Autodesk Fusion 360 part; units mm, degrees
sketch "スケッチ1" plane through (0, 0, 0) normal (0, 0, 1) x (1, 0, 0)
  line L0 (0, 0) -> (18.0857, 0)
  line L1 (18.0857, 0) -> (18.0857, 13.2439)
  line L2 (18.0857, 13.2439) -> (0, 13.2439)
  line L3 (0, 13.2439) -> (0, 0)
  line L4 (0, 0) -> (-13.9996, 0)
  line L5 (-13.9996, 0) -> (-13.9996, 13.2439)
  line L6 (-13.9996, 13.2439) -> (0, 13.2439)
  line L7 (0, 13.2439) -> (0, 0)
  circle A0 centre (-6.9857, 4.9) radius 2
  circle A1 centre (6.9857, 4.9) radius 2
  circle A2 centre (0, 9) radius 2
  circle A3 centre (14.1857, 2.8) radius 3
  circle A4 centre (-6.9857, 4.9) radius 2.5
  circle A5 centre (6.9857, 4.9) radius 2.5
  circle A6 centre (0, 9) radius 2.3
  circle A7 centre (0, 9) radius 1.7
  line L8 (-7, 1.5) -> (-7, 0)
  line L9 (7, 1.5) -> (7, 0)
  circle A8 centre (-6.9857, 4.9) radius 3.4
  circle A9 centre (0, 9) radius 2.9
  line L10 (-6.9857, 4.9) -> (0, 9)
  line L11 (0, 9) -> (6.9857, 4.9)
  line L12 (6.9857, 4.9) -> (14.1857, 2.8)
  circle A10 centre (6.9857, 4.9) radius 3.4
  circle A11 centre (14.1857, 2.8) radius 3.9
  line L13 (-4.6, 2.4775) -> (-4.6, 0)
  line L14 (4.6, 2.4775) -> (4.6, 0)
  line L15 (-9.4, 2.506) -> (-9.4, 0)
  line L16 (9.4, 2.506) -> (9.4, 0)
  line L17 (-3.6347, 5.4753) -> (-1.6695, 6.6287)
  line L18 (1.6695, 6.6287) -> (3.6347, 5.4753)
  line L19 (-4.8495, 7.5452) -> (-2.8843, 8.6986)
  line L20 (2.8843, 8.6986) -> (4.8495, 7.5452)
  line L21 (10.2588, 5.8204) -> (11.3683, 5.4967)
  line L22 (9.2508, 2.3644) -> (10.3603, 2.0407)
  line L23 (0, 0) -> (18.0857, 0)
  line L24 (18.0857, 0) -> (18.0857, -2.0683)
  line L25 (18.0857, -2.0683) -> (0, -2.0683)
  line L26 (-13.9996, 0) -> (0, 0)
  line L27 (0, -2.0683) -> (-13.9996, -2.0683)
  line L28 (-13.9996, -2.0683) -> (-13.9996, 0)
  line L29 (-12.3, 6.4) -> (-12.3, 10)
  line L30 (-12.3, 10) -> (-8.7, 10)
  line L31 (-8.7, 10) -> (-8.7, 7.8362)
  line L32 (-12.3, 6.4) -> (-10.0369, 6.4)
  line L33 (-5.5, 1.65) -> (-8.5, 1.65)
  line L34 (-8.5, 1.65) -> (-8.5, 0.4)
  line L35 (-8.5, 0.4) -> (-5.5, 0.4)
  line L36 (-5.5, 0.4) -> (-5.5, 1.65)
  line L37 (-5.5, 1.65) -> (-8.5, 0.4) construction
  line L38 (-8.5, 1.65) -> (-5.5, 0.4) construction
  line L39 (8.5, 1.65) -> (5.5, 1.65)
  line L40 (5.5, 1.65) -> (5.5, 0.4)
  line L41 (5.5, 0.4) -> (8.5, 0.4)
  line L42 (8.5, 0.4) -> (8.5, 1.65)
  line L43 (8.5, 1.65) -> (5.5, 0.4) construction
  line L44 (5.5, 1.65) -> (8.5, 0.4) construction
  arc A12 (-12.3, 9.4) -> (-9.3, 6.4) centre (-9.3, 9.4) ccw
  point P0 (-7, 1.5)
  point P1 (7, 1.5)
  point P2 (-10.5, 10)
  point P3 (-7, 1.025)
  point P4 (7, 1.025)
  dimension "d4" = 4
  dimension "d5" = 4.9
  dimension "d6" = 8.1
  dimension "d7" = 4
  dimension "d10" = 6
  dimension "d16" = 2.8
  dimension "d18" = 9
  dimension "d19" = 5
  dimension "d21" = 7.5
  dimension "d26" = 4.6
  dimension "d34" = 3.4
  dimension "d41" = 7
  dimension "d45" = 5.8
  dimension "d51" = 1.2
  dimension "d52" = 4.8
  dimension "d54" = 1.8
  dimension "d57" = 6.8
  dimension "d76" = 7.8
  dimension "d86" = 10.5
  dimension "d87" = 3.6
  dimension "d88" = 10
  dimension "d92" = 3
  dimension "d93" = 0.4
  dimension "d94" = 1.25
  dimension "d96" = 3.6
  dimension "d97" = 3
extrude "押し出し1" add sketch "スケッチ1" along normal blind 3 contours L0 L9 A10 L14 L23 L39 L40 L41 | L3 L7 A6 A9 L10 | L3 L7 A6 A9 L11 | L4 L8 A8 L13 L26 L33 L35 L36 | L0 L9 A10 L16 L22 L23 L39 L41 L42 | A5 L11 L12 A10 L39 | A8 A9 L10 L17 | A9 L11 A10 L18 | L4 L8 A8 L15 L26 L33 L34 L35 | A8 L33 | L3 L7 A6 A9 L10 | L3 L7 A6 A9 L11 | A8 A9 L10 L19 | A9 L11 A10 L20 | L0 A3 L12 A11 L23 | L0 A3 A11 L23 | A10 L16 L22 | L12 A10 A11 L16 L22 | A5 L11 L12 A10 | L0 A3 L12 A11 L23 | L12 A10 A11 L21 | A8 L29 L30 L31 A12 picked at (-7.0288, 1.9011)
extrude "押し出し2" add sketch "スケッチ1" along normal blind 0.5 contours A4 | A1 A5 L11 L12 | A1 A5 L11 L12
extrude "押し出し5" add sketch "スケッチ1" against normal blind 2.3 from surface at 3 contours L3 L7 A2 A6 L10 | L3 L7 A2 A6 L11 | L3 L7 A2 A6 L10 | L3 L7 A2 A6 L11
sketch "スケッチ2" plane through (0, 0, 0) normal (0, -1, 0) x (1, 0, 0)
  line L0 (-7, 0) -> (-7, 3)
  line L1 (7, 0) -> (7, 3)
  circle A0 centre (-7, 1.5) radius 0.8
  circle A1 centre (7, 1.5) radius 0.8
  line L2 (9.4, 0) -> (9.4, 3)
  line L3 (4.6, 3) -> (4.6, 0)
  line L4 (-4.6, 3) -> (-9.4, 3)
  line L5 (4.6, 0) -> (9.4, 0)
  line L6 (-4.6, 0) -> (-4.6, 3)
  line L7 (-9.4, 3) -> (-9.4, 0)
  line L8 (9.4, 3) -> (4.6, 3)
  line L9 (-9.4, 0) -> (-4.6, 0)
  point P0 (7, 0)
  dimension "d42" = 1.6
extrude "押し出し7" cut sketch "スケッチ2" against normal blind 3 contours L0 A0 | L0 A0 | L1 A1 | L1 A1
extrude "押し出し8" add sketch "スケッチ1" against normal blind 0.3 from surface at 1 contours L3 L7 A2 A7 L10 | L3 L7 A2 A7 L11 | L3 L7 A2 A7 L10 | L3 L7 A2 A7 L11
sketch "スケッチ6" plane through (0, 10, 0) normal (0, 1, 0) x (-1, 0, 0)
  line L0 (8.7, 0) -> (12.3, 0)
  line L1 (12.3, 0) -> (12.3, 3)
  line L2 (12.3, 3) -> (8.7, 3)
  line L3 (8.7, 3) -> (8.7, 0)
  line L4 (10.5, 3) -> (10.5, 0)
  circle A0 centre (10.5, 1.5) radius 0.75
  dimension "d89" = 1.5
extrude "押し出し12" cut sketch "スケッチ6" against normal blind 2.6 contours L4 A0 | L4 A0
equation "d5 = 6.5 mm - 0.6 mm - 1.0 mm"
equation "d6 = 6 mm + 2.0 mm + 0.1 mm"
equation "d16 = ( 7.8 / 2 ) * 1 mm - 0.6 mm - 0.5 mm"
equation "d21 = 6 mm + 1.4 mm + 0.1 mm"
Input: part model. Units: mm. Frame: model coordinates. A direction names the side the tool comes from. Coordinates: 2 decimals unless noted, no trailing zeros. Write each loop counter-clockwise with the first axis right and the second up, starting at its lowest first coordinate (ties: lowest second). Pieces come first, ordered by that corner, then holes.
1) Pin query (flat end, axial travel): pin 1 Ø1.4 at (y, z) = (1, 1) entering from +X; pin 2 Ø6.5 at (x, y) = (6.99, 4.9) entering from -Z; pin 3 Ø0.7 at (x, z) = (8, 1.5) entering from -Y; pin 4 Ø1.2 at (x, z) = (8, 2) entering from +Y. Return the tip coordinate at first contact, or that it passes through.
2) Set-up query: faces 4 (the cylindrical face through (7.739, 2.087, 1.194)), 5 (the cylindrical face through (0, 11, 2)), 6 (the flat face through (9.4, 1, 1)), 7 (the flat face through (5.5, 1, 1)), 8 (the flat face through (-10.5, 7.4, 1.5)). Return all of +Z, -Z, +X, -X, +Y, -Y with unobstructed straight access to the full face (end or side cutting, diameter ignored); none if empty.
3) Mould query, pull axis X, two halves, no side actions, for faces 1 (the flat face through (-11.33, 10, 1.15)), 2 (the cylindrical face through (-6.758, 8.292, 1.479)), 3 (the flat face through (-9.4, 1, 1)). Classes: pulls with the +X half, pulls with the -X half, needs draft (parallel to the pull), parting line crosses it, or undercut.
4) Section A-A on x = -1. Output: boundary loops of the cut face in (y, z), and give its area (3 significant figures).
5) Section B-B on z = 1.5. State how many separate pieces and enclosed holes the cut face has, and give its area (3 significant figures).
6) Material intervals for line 1 along X through (y, z) = (6, 2.8); line 2 along X through (y, z) = (4.9, 2); line 3 along Z through (x, y) = (7, 2.3), sorted ascending.
Check result:
1. pin 1: stops at x = 17.93
1. pin 2: stops at z = 0
1. pin 3: stops at y = 0
1. pin 4: stops at y = 8.27
2. face 4: -Y
2. face 5: +Z
2. face 6: +Z, -Z, -Y
2. face 7: +Z, -Z
2. face 8: +Y
3. face 1: needs draft
3. face 2: undercut
3. face 3: pulls with the -X half
4. outline: (6.28, 0) - (6.93, 0) - (6.93, 0.7) - (7.63, 0.7) - (7.63, 1) - (7.27, 1) - (7.27, 3) - (6.28, 3) - close; (10.37, 0.7) - (11.07, 0.7) - (11.07, 0) - (11.72, 0) - (11.72, 3) - (10.73, 3) - (10.73, 1) - (10.37, 1) - close
4. area: 5.68 mm2
5. separate pieces: 1
5. enclosed holes: 2
5. area: 90.0 mm2
6. line 1: x = -10.2 to -9.23, -4.74 to -2.74, 2.74 to 4.74, 9.23 to 10.2, 11.96 to 16.42
6. line 2: x = -10.39 to -9.49, -4.49 to -3.59, 3.59 to 4.49, 9.49 to 12.04, 16.33 to 17.47
6. line 3: z = 0 to 0.7, 2.3 to 3
